Geometry check sheet. Reference: the model listing, model coordinates, mm. Round coordinates to 2 decimals unless told otherwise and drop trailing zeros. Write each loop counter-clockwise with the first axis right and the second up, starting at its lowest first coordinate (ties: lowest second). Pieces come first, ordered by that corner, then holes.
Item 1: Cross-section at D-D (x = 3). Enter the section's corners in (y, z).
Item 2: Cross-section at C-C (x = 10). Enter the section's corners in (y, z), then the cut area to 3 significant figures.
Item 3: Scan lines: probe 1 along Z at (x, y) = (10, 14); probe 2 along X at (y, z) = (8.5, 88.5); probe 3 along Z at (x, y) = (10.5, 16). Record each from-to range of solid material in increasing order.
Item 4: Depth check by flat-ended pin: P1, Ø4, axis at x = 2.5, y = 11, coming from the -Z side; P2, Ø4, axis at y = 6.5, z = 45, coming from the -X side; P3, Ø4, axis at y = 11, z = 131, coming from the +X side; P4, Ø8, axis at x = 5.5, y = 3.5, coming from the +Z side. Enter the tip coordinate at first touch or a pass-through.
Item 5: Cross-section at B-B (y = 1.75). Enter the section's corners in (x, z), then the cut area to 3 significant figures.
Item 6: Cross-section at A-A (z = 20). Enter the section's corners in (x, y), then the cut area to 3 significant figures.
from build123d import *

# Parameters (mm, degrees)
SKETCH_1_W               = 20
SKETCH_1_H               = 20
EXTRUDE_1_DEPTH          = 154.23
CUT_EXTRUDE_1_DEPTH      = 154.23
CUT_EXTRUDE_2_DEPTH      = 157.802081938
CUT_EXTRUDE_2_DEPTH_BACK = 157.802081938
SKETCH_3_R               = 2


with BuildPart() as part:
    # 草图1 → 凸台-拉伸1 (new body)
    with BuildSketch(Plane.XY):
        with Locations((10, 10)):
            Rectangle(SKETCH_1_W, SKETCH_1_H)
    extrude(amount=EXTRUDE_1_DEPTH)

    # 草图2 → 切除-拉伸1 (cut)
    with BuildSketch(Plane(origin=(0, 20, 0), x_dir=(1, 0, 0), z_dir=(0, 1, 0))):
        Polygon((0, -154.23), (20, -119.588983849), (20, -154.23), align=None)
        Polygon((20, -11.547005384), (0, 0), (20, 0), align=None)
    extrude(amount=-CUT_EXTRUDE_1_DEPTH, mode=Mode.SUBTRACT)

    # 草图3 → 切除-拉伸2 (cut, two sides: drawn at the far end of the back side and taken through both)
    with BuildSketch(Plane(origin=(0, 20, 0), x_dir=(1, 0, 0), z_dir=(0, 1, 0)).offset(-CUT_EXTRUDE_2_DEPTH_BACK)):
        with Locations(Location((10, -88.5, 0), (0, 0, 270))):
            Circle(SKETCH_3_R)
        with Locations(Location((10, -118.5, 0), (0, 0, 270))):
            Circle(SKETCH_3_R)
        with Locations(Location((10, -58.5, 0), (0, 0, 270))):
            Circle(SKETCH_3_R)
        with Locations(Location((10, -20, 0), (0, 0, 270))):
            Circle(SKETCH_3_R)
        with Locations(Location((10, -40, 0), (0, 0, 270))):
            Circle(SKETCH_3_R)
    extrude(amount=CUT_EXTRUDE_2_DEPTH + CUT_EXTRUDE_2_DEPTH_BACK, mode=Mode.SUBTRACT)


solid = part.part
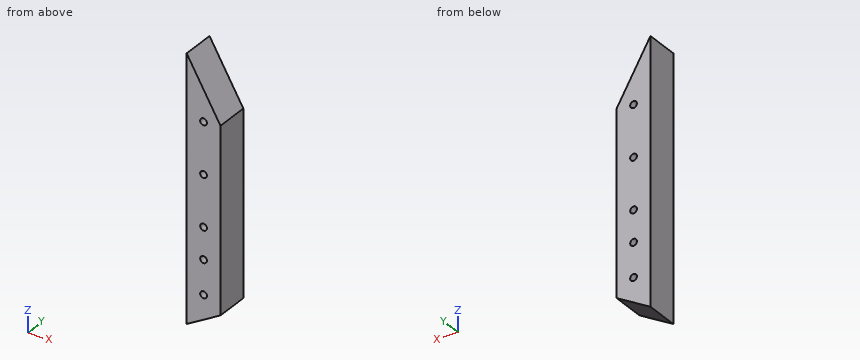
Resolved:
1. outline: (0, 1.73) - (20, 1.73) - (20, 149.03) - (0, 149.03) - close
2. outline: (0, 5.77) - (20, 5.77) - (20, 18) - (0, 18) - close; (0, 22) - (20, 22) - (20, 38) - (0, 38) - close; (0, 42) - (20, 42) - (20, 56.5) - (0, 56.5) - close; (0, 60.5) - (20, 60.5) - (20, 86.5) - (0, 86.5) - close; (0, 90.5) - (20, 90.5) - (20, 116.5) - (0, 116.5) - close; (0, 120.5) - (20, 120.5) - (20, 136.91) - (0, 136.91) - close
2. area: 2,220 mm2
3. probe 1: z = 5.77 to 18, 22 to 38, 42 to 56.5, 60.5 to 86.5, 90.5 to 116.5, 120.5 to 136.91
3. probe 2: x = 0 to 8, 12 to 20
3. probe 3: z = 6.06 to 18.06, 21.94 to 38.06, 41.94 to 56.56, 60.44 to 86.56, 90.44 to 116.56, 120.44 to 136.04
4. P1: stops at z = 0.29
4. P2: stops at x = 0
4. P3: stops at x = 14.57
4. P4: stops at z = 151.63
5. outline: (0, 0) - (20, 11.55) - (20, 119.59) - (0, 154.23) - close; hole circle Ø4 at (10, 20); hole circle Ø4 at (10, 40); hole circle Ø4 at (10, 58.5); hole circle Ø4 at (10, 88.5); hole circle Ø4 at (10, 118.5)
5. area: 2,560 mm2
6. outline: (0, 0) - (8, 0) - (8, 20) - (0, 20) - close; (12, 0) - (20, 0) - (20, 20) - (12, 20) - close
6. area: 320 mm2
